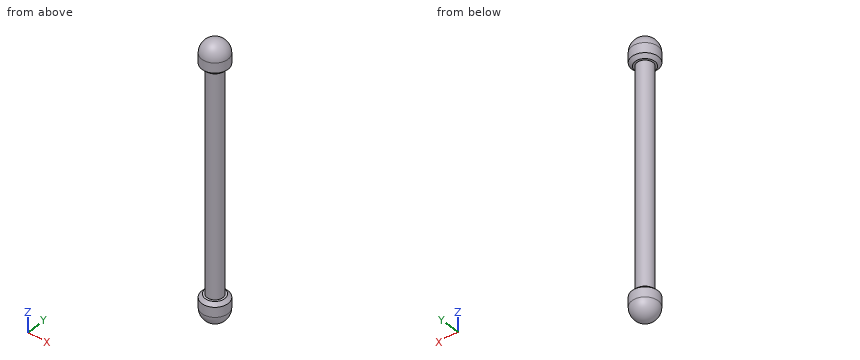
```python
from build123d import *

# Parameters (mm, degrees)
F0_R     = 4.8
F1_DEPTH = 136
F2_R     = 8
F3_DEPTH = 16
F4_R     = 8
F5_DEPTH = 16
F6_R     = 8
F7_SIZE  = 2


with BuildPart() as f1:
    # F0 (on Top) → F1 (new body)
    with BuildSketch(Plane.XY):
        Circle(F0_R)
    extrude(amount=F1_DEPTH)

    # F2 (on face) → F3 (join)
    with BuildSketch(Plane(origin=(0, 0, 0), x_dir=(1, 0, 0), z_dir=(0, 0, -1))):
        Circle(F2_R)
    extrude(amount=F3_DEPTH)

    # F4 (on face) → F5 (join)
    with BuildSketch(Plane.XY.offset(136)):
        Circle(F4_R)
    extrude(amount=F5_DEPTH)

    # F6
    f6_edges = [f1.edges().sort_by_distance(p)[0] for p in [
        (-8, 0, -16),
        (-8, 0, 152),
    ]]
    fillet(f6_edges, radius=F6_R)

    # F7
    f7_edges = [f1.edges().sort_by_distance(p)[0] for p in [
        (-8, 0, 0),
        (-8, 0, 136),
    ]]
    chamfer(f7_edges, length=F7_SIZE)


solid = f1.part
```
The listing builds one solid part. Answer for the finished solid, in the listing's coordinates (mm). Coordinates: 2 decimals unless noted, no trailing zeros. Write each loop counter-clockwise with the first axis right and the second up, starting at its lowest first coordinate (ties: lowest second). Pieces come first, ordered by that corner, then holes. Notation, with made-up numbers: (40, 35.5) - (55, 35.5) arc R22 cw to (55, 46.5) - close; hole circle Ø9 at (49, -31). An arc over 180 degrees is marked (long way). Return JSON: item names as keys, results as strings. Group by question number.
Q1. The part is cut by section A-A on x = 0. Write down the section's boundary in (y, z).
Q2. Find the intervals of material crossed by line 1 along Z through (x, y) = (2, 5); line 2 along X through (y, z) = (0.5, 39.5); line 3 along Z through (x, y) = (4.25, 5.5), in increasing order. Write a range as [from, to].
Q3. The part is cut by section C-C on z = 73. Write down the section's boundary in (x, y).
Q4. Flat-ended cylindrical pins translate along their axes: pin 1 Ø4 at (x, y) = (-5, 4) entering from +Z; pin 2 Ø6 at (x, z) = (1, 12) entering from +Y; pin 3 Ø1.5 at (x, y) = (-1.5, -4.5) entering from +Z. Find the tip coordinate at first contact, or state that the pin passes through.
Evaluation:
{
 "1": {"outline": "(-8, -8) arc R8 ccw to (8, -8) - (8, -2) - (6, 0) - (4.8, 0) - (4.8, 136) - (6, 136) - (8, 138) - (8, 144) arc R8 ccw to (-8, 144) - (-8, 138) - (-6, 136) - (-4.8, 136) - (-4.8, 0) - (-6, 0) - (-8, -2) - close"},
 "2": {"line 1": "z = [-13.92, 0], [136, 149.92]", "line 2": "x = [-4.77, 4.77]", "line 3": "z = [-11.96, -0.95], [136.95, 147.96]"},
 "3": {"outline": "circle Ø9.6 at (0, 0)"},
 "4": {"pin 1": "stops at z = 150.68", "pin 2": "stops at y = 4.8", "pin 3": "stops at z = 150.93"}
}
